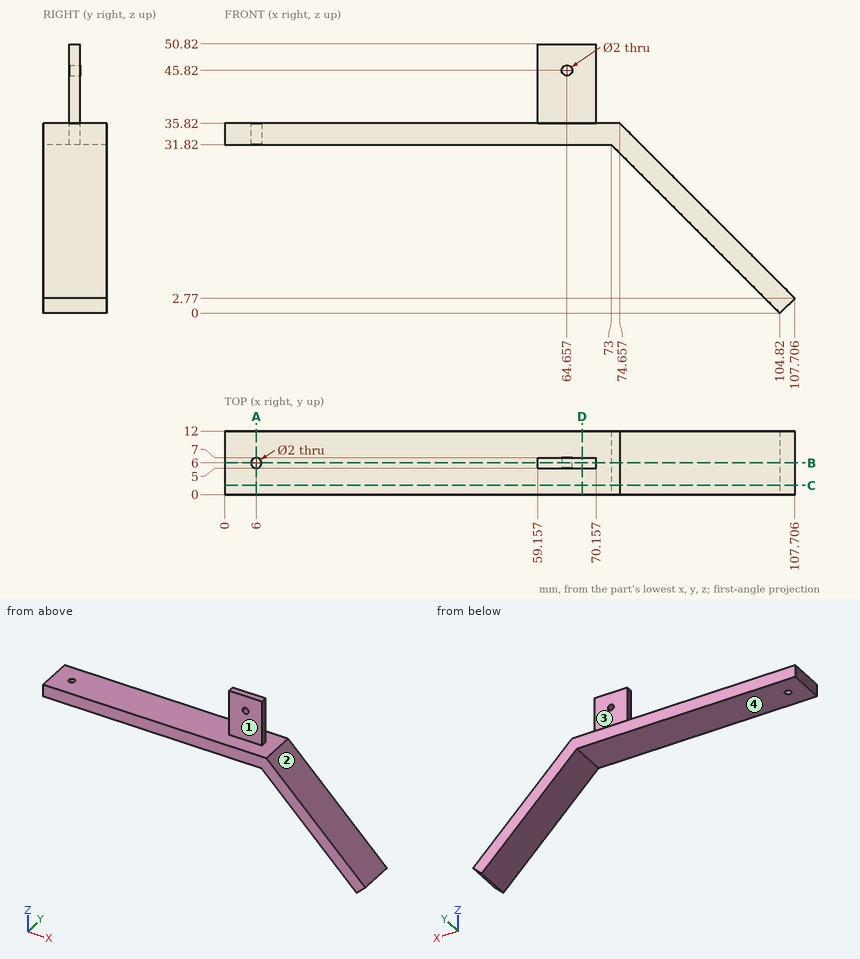
Drawing for the job (mm, zero at the part's lowest x, y, z). A direction names the side the tool comes from. Round coordinates to 2 decimals unless told otherwise and drop trailing zeros. Order: outer loops, then holes, each group sorted by start corner. A loop starts at its lowest first (then second) coordinate and runs counter-clockwise, first axis right, second up. Notation, with made-up numbers: (-23.75, -22) -> (-10.75, -22) arc R17 cw to (-10.75, -13) -> close; hole circle Ø7 at (31.5, -8.5). An arc over 180 degrees is marked (long way). Put each result on its own line as item: value.
Q1. Pin check, flat tips, straight feed: pin 1 Ø5 at (x, y) = (62, 2.5) entering from -Z; pin 2 Ø4 at (y, z) = (9, 16.5) entering from -X; pin 3 Ø3 at (y, z) = (7, 17.5) entering from +X; pin 4 Ø8 at (x, z) = (74.5, 19.5) entering from -Y. Stop position of each tip, or through.
From the geometry:
pin 1: stops at z = 31.82
pin 2: stops at x = 86.32
pin 3: stops at x = 94.48
pin 4: passes through
Q2. Band-saw the part on C-C (y = 1.75). Give the cut face in (x, z), and give its area (3 significant figures).
From the geometry:
outline: (0, 31.82) -> (73, 31.82) -> (104.82, 0) -> (107.71, 2.77) -> (74.66, 35.82) -> (0, 35.82) -> close
area: 479 mm2
Q3. Band-saw the part on D-D (x = 67.5). Give the cut face in (y, z), and give its area (3 significant figures).
From the geometry:
outline: (0, 31.82) -> (12, 31.82) -> (12, 35.82) -> (7, 35.82) -> (7, 50.82) -> (5, 50.82) -> (5, 35.82) -> (0, 35.82) -> close
area: 78.0 mm2
Q4. Band-saw the part on B-B (y = 6). Give the cut face in (x, z).
From the geometry:
outline: (0, 31.82) -> (5, 31.82) -> (5, 35.82) -> (0, 35.82) -> close; (7, 31.82) -> (73, 31.82) -> (104.82, 0) -> (107.71, 2.77) -> (74.66, 35.82) -> (70.16, 35.82) -> (70.16, 50.82) -> (59.16, 50.82) -> (59.16, 35.82) -> (7, 35.82) -> close; hole circle Ø2 at (64.66, 45.82)
Q5. Wall check: line 1 (Y direction, x = 6, z = 34.9); line 2 (Z direction, x = 18, y = 8.5); line 3 (X direction, y = 3.5, z = 22) (1 decimal). Give the ranges that are in metal, low to high. Write a range as [from, to].
From the geometry:
line 1: y = [0, 5], [7, 12]
line 2: z = [31.82, 35.82]
line 3: x = [82.8, 88.5]
Q6. Band-saw the part on A-A (x = 6). Give the cut face in (y, z), and give its area (3 significant figures).
From the geometry:
outline: (0, 31.82) -> (5, 31.82) -> (5, 35.82) -> (0, 35.82) -> close; (7, 31.82) -> (12, 31.82) -> (12, 35.82) -> (7, 35.82) -> close
area: 40.0 mm2
Q7. Tool access for the marked faces 1, 2, 3 and 4: list every direction of +Z, -Z, +X, -X, +Y, -Y with a clear straight run to the whole face (end or side of a thin tool).
From the geometry:
face 1: +Z, +X, -X, -Y
face 2: +Z, +X, +Y, -Y
face 3: +Z, +X, -X, +Y
face 4: -Z, -X, +Y, -Y
